Geometry check sheet. Reference: the model listing, model coordinates, mm. Face numbers are marked on the shaded views. A direction names the side the tool comes from. Round coordinates to 2 decimals unless told otherwise and drop trailing zeros. Order: outer loops, then holes, each group sorted by start corner. A loop starts at its lowest first (then second) coordinate and runs counter-clockwise, first axis right, second up. Notation, with made-up numbers: (66, 49.5) -> (78, 49.5) arc R33 cw to (78, 78.5) -> close; hole circle Ø7 at (44, 19). An arc over 180 degrees is marked (long way). Use a Markdown table: item, result. Add a question column.
Item 1: Sectioned sample at C-C, the plane z = 181. Record the cut outline in (x, y).
Item 2: Mould release check, pull along Y, two halves, no side actions. Record for the marked faces 3, 4 and 5: pulls with the +Y half, pulls with the -Y half, needs draft (parallel to the pull), parting line crosses it, or undercut.
Item 3: Material ranges on probe 1 along Z at (x, y) = (214, 58); probe 2 along X at (y, z) = (9, 84); probe 3 along X at (y, z) = (46.5, 194), recorded low to high. Write a range as [from, to].
Item 4: Sectioned sample at B-B, the plane x = 224. Record the cut outline in (y, z).
Item 5: Gauge pin test, flat ends, axial feed: pin 1 Ø1.5 at (y, z) = (60, 120) entering from +X; pin 2 Ø8 at (x, y) = (91.5, 57) entering from +Z; pin 3 Ø2.5 at (x, z) = (260.01, 161.4) entering from -Y. Record the tip position at first contact, or that the pin passes through.
Item 6: Sectioned sample at A-A, the plane y = 61.5. Record the cut outline in (x, z).
Item 7: Set-up check for the marked faces 1 and 2: record each of +Z, -Z, +X, -X, +Y, -Y from which the full face is reachable in a straight line by a thin tool's end or side.
Item 8: Sectioned sample at D-D, the plane y = 29.5. Record the cut outline in (x, z), and give its area (3 significant figures).
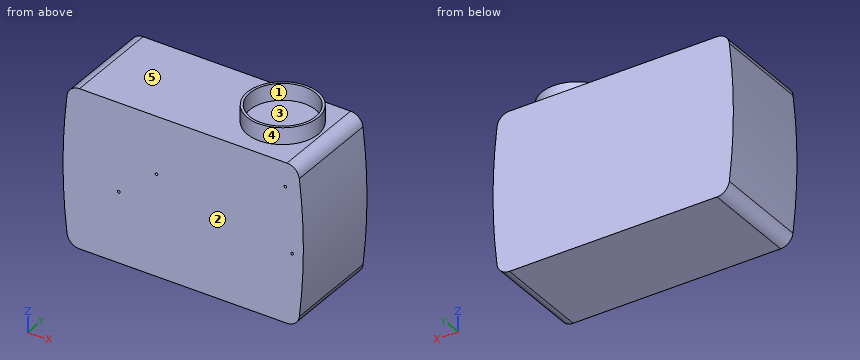
from build123d import *

# Parameters (mm, degrees)
F1_DEPTH = 115
F2_D     = 3.2
F2_DEPTH = 20
F2_TIP   = 0.9613769904
F3_R     = 42.5
F3_R_2   = 39.5
F4_DEPTH = 20


with BuildPart() as f1:
    # F0 (on Front) → F1 (new body)
    with BuildSketch(Plane.XZ):
        with BuildLine():
            ThreePointArc((-1.6878500476, 13.2459854015), (3.2420540262, 3.7904010112), (13.2092447292, 0))
            Line((13.2092447292, 0), (261.8105676743, 0))
            ThreePointArc((261.8105676743, 0), (271.7777583774, 3.7904010112), (276.7076624511, 13.2459854015))
            ThreePointArc((276.7076624511, 13.2459854015), (281.5099062018, 95.1), (276.7076624511, 176.9540145985))
            ThreePointArc((276.7076624511, 176.9540145985), (271.7777583774, 186.4095989888), (261.8105676743, 190.2))
            Line((261.8105676743, 190.2), (13.2092447292, 190.2))
            ThreePointArc((13.2092447292, 190.2), (3.2420540262, 186.4095989888), (-1.6878500476, 176.9540145985))
            ThreePointArc((-1.6878500476, 176.9540145985), (-6.4900937982, 95.1), (-1.6878500476, 13.2459854015))
        make_face()
    extrude(amount=-F1_DEPTH)

    # F2
    with Locations(Plane.XZ):
        with Locations((60.4099062018, 84.4), (105.5099062018, 121.4), (268.0099062018, 84.9), (260.0099062018, 161.4)):
            Hole(F2_D / 2, depth=F2_DEPTH)
            with Locations((0, 0, -(F2_DEPTH + F2_TIP / 2))):  # 118° drill point
                Cone(0, F2_D / 2, F2_TIP, mode=Mode.SUBTRACT)

    # F3 (on face) → F4 (join)
    with BuildSketch(Plane.XY.offset(190.2)):
        with Locations((216.0099062018, 61.5)):
            Circle(F3_R)
        with Locations((216.0099062018, 61.5)):
            Circle(F3_R_2, mode=Mode.SUBTRACT)
    extrude(amount=F4_DEPTH)


solid = f1.part
Found:
| question | item | result |
|---|---|---|
| 1 | outline | (-0.62, 0) -> (275.64, 0) -> (275.64, 115) -> (-0.62, 115) -> close |
| 2 | face 3 | undercut |
| 2 | face 4 | parting line crosses it |
| 2 | face 5 | needs draft |
| 3 | probe 1 | z = [0, 190.2] |
| 3 | probe 2 | x = [-6.4, 58.86], [61.96, 266.69], [269.33, 281.42] |
| 3 | probe 3 | x = [176.24, 179.47], [252.55, 255.77] |
| 4 | outline | (0, 0) -> (115, 0) -> (115, 190.2) -> (103.24, 190.2) -> (103.24, 210.2) -> (100.18, 210.2) -> (100.18, 190.2) -> (22.82, 190.2) -> (22.82, 210.2) -> (19.76, 210.2) -> (19.76, 190.2) -> (0, 190.2) -> close |
| 5 | pin 1 | stops at x = 281.09 |
| 5 | pin 2 | stops at z = 190.2 |
| 5 | pin 3 | stops at y = 20.21 |
| 6 | outline | (-1.69, 13.25) arc R15 ccw to (13.21, 0) -> (261.81, 0) arc R15 ccw to (276.71, 13.25) arc R700 ccw to (276.71, 176.95) arc R15 ccw to (261.81, 190.2) -> (258.51, 190.2) -> (258.51, 210.2) -> (255.51, 210.2) -> (255.51, 190.2) -> (176.51, 190.2) -> (176.51, 210.2) -> (173.51, 210.2) -> (173.51, 190.2) -> (13.21, 190.2) arc R15 ccw to (-1.69, 176.95) arc R700 ccw to start |
| 7 | face 1 | +Z |
| 7 | face 2 | +Z, -Z, +X, -X, -Y |
| 8 | outline | (-1.69, 13.25) arc R15 ccw to (13.21, 0) -> (261.81, 0) arc R15 ccw to (276.71, 13.25) arc R700 ccw to (276.71, 176.95) arc R15 ccw to (261.81, 190.2) -> (243.98, 190.2) -> (243.98, 210.2) -> (239.17, 210.2) -> (239.17, 190.2) -> (192.85, 190.2) -> (192.85, 210.2) -> (188.04, 210.2) -> (188.04, 190.2) -> (13.21, 190.2) arc R15 ccw to (-1.69, 176.95) arc R700 ccw to start |
| 8 | area | 54,000 mm2 |
